Study the drawing (mm; zero at the part's minimum x, y, z) and answer. Round coordinates to 2 decimals unless told otherwise and drop trailing zeros. Loops run counter-clockwise (first coordinate to the right, second up) from the corner with the lowest first, then second, coordinate; pieces in that order, holes last. Notation, with made-up numbers: (44.5, 15.25) - (86.5, 15.25) arc R21 cw to (86.5, 43.25) - close; hole circle Ø1 at (-19, 62). An arc over 180 degrees is marked (long way). Use CSV: the item, a comma, the result in double quotes. Start each with the question number.
1. Find section B-B (z = 38). Give the vertices of the cut face in (x, y).
2. Find section A-A (y = 0.6). Give the vertices of the cut face in (x, z), and give its area (3 significant figures).
3. Find section C-C (x = 176). Give the vertices of the cut face in (y, z).
4. Consider line 1 along Z through (x, y) = (368, 1.15); line 2 along X through (y, z) = (0.7, 20); line 3 along Z through (x, y) = (186, 0.85). Determine where each line is inside the solid, lowest interval first.
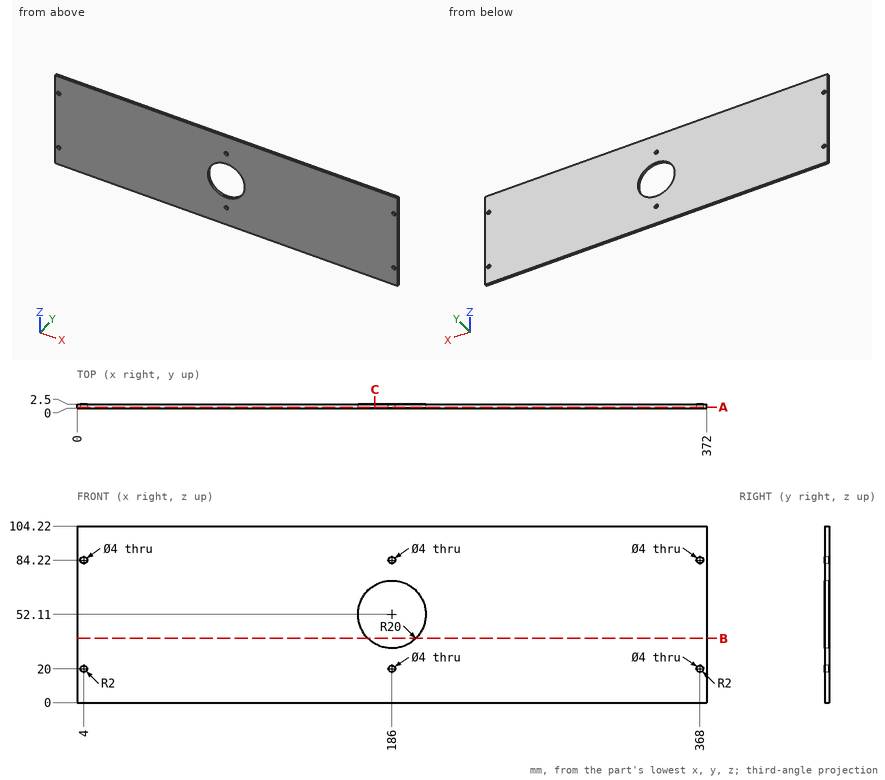
Filled sheet:
1,outline,"(0, 0) - (171.83, 0) - (171.83, 2.5) - (0, 2.5) - close; (200.17, 0) - (372, 0) - (372, 2.5) - (200.17, 2.5) - close"
2,outline,"(0, 0) - (372, 0) - (372, 104.22) - (0, 104.22) - close; hole circle Ø4 at (4, 20); hole circle Ø4 at (4, 84.22); hole circle Ø40 at (186, 52.11); hole circle Ø4 at (186, 20); hole circle Ø4 at (186, 84.22); hole circle Ø4 at (368, 20); hole circle Ø4 at (368, 84.22)"
2,area,"37,400 mm²"
3,outline,"(0, 0) - (2.5, 0) - (2.5, 34.79) - (0, 34.79) - close; (0, 69.43) - (2.5, 69.43) - (2.5, 104.22) - (0, 104.22) - close"
4,line 1,"z = 0 to 18, 22 to 82.22, 86.22 to 104.22"
4,line 2,"x = 0 to 2, 6 to 184, 188 to 366, 370 to 372"
4,line 3,"z = 0 to 18, 22 to 32.11, 72.11 to 82.22, 86.22 to 104.22"
